Model file for the job. Use its own axes, mm. Face numbers are marked on the shaded views. A direction names the side the tool comes from. Round coordinates to 2 decimals unless told otherwise and drop trailing zeros. Order: outer loops, then holes, each group sorted by start corner. A loop starts at its lowest first (then second) coordinate and runs counter-clockwise, first axis right, second up. Notation, with made-up numbers: (6.25, 82) - (44.25, 82) arc R19 cw to (44.25, 109) - close; hole circle Ø11 at (7.5, 6.5). An arc over 180 degrees is marked (long way). Use one line per item in the form item = value.
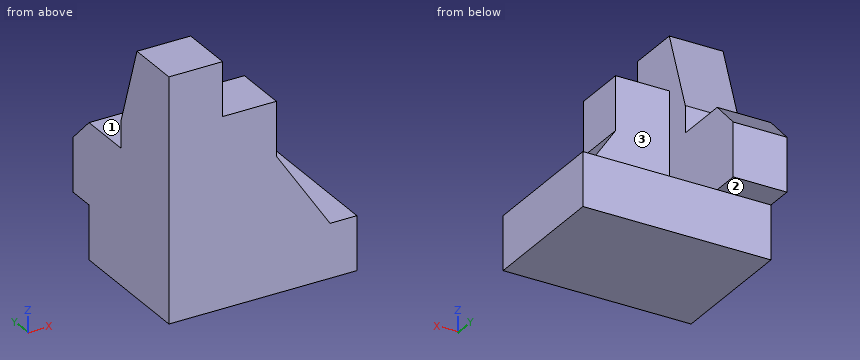
from build123d import *

# Parameters (mm, degrees)
BOSS_EXTRUDE1_DEPTH = 2
BOSS_EXTRUDE2_DEPTH = 3
SKETCH3_W           = 2
SKETCH3_H           = 3
BOSS_EXTRUDE3_DEPTH = 1
CUT_EXTRUDE1_DEPTH  = 3


with BuildPart() as part:
    # Sketch1 → Boss-Extrude1 (new body)
    with BuildSketch(Plane(origin=(0, 0, 0), x_dir=(1, 0, 0), z_dir=(0, 1, 0))):
        Polygon((0, 0), (2, 0), (2, 2), (4, 2), (4, 4), (6, 7), (7, 7), (7, 9), (0, 9), align=None)
    extrude(amount=BOSS_EXTRUDE1_DEPTH)

    # Sketch2 → Boss-Extrude2 (add)
    with BuildSketch(Plane(origin=(0, 2, 0), x_dir=(1, 0, 0), z_dir=(0, 1, 0))):
        Polygon((7, 9), (0, 9), (0, 0), (2, 0), (2, 7), (7, 7), align=None)
    extrude(amount=BOSS_EXTRUDE2_DEPTH)

    # Sketch3 → Boss-Extrude3 (add)
    with BuildSketch(Plane(origin=(0, 5, 0), x_dir=(1, 0, 0), z_dir=(0, 1, 0))):
        with Locations((1, 5.5)):
            Rectangle(SKETCH3_W, SKETCH3_H)
    extrude(amount=BOSS_EXTRUDE3_DEPTH)

    # Sketch4 → Cut-Extrude1 (cut, through all)
    with BuildSketch(Plane(origin=(2, 0, 0), x_dir=(0, 0, -1), z_dir=(1, 0, 0))):
        Polygon((4, 5), (5, 6), (4, 6), align=None)
        Polygon((4, 3), (4, 5), (0, 5), (0, 2), (3, 3), align=None)
    extrude(amount=-CUT_EXTRUDE1_DEPTH, mode=Mode.SUBTRACT)


solid = part.part
(1) Slice it at B-B on x = 2.75. Give the cut face in (y, z).
Report:
outline = (0, -9) - (5, -9) - (5, -7) - (2, -7) - (2, -2) - (0, -2) - close
(2) Slice it at A-A on y = 0.85. Give the cut face in (x, z).
Report:
outline = (0, -9) - (7, -9) - (7, -7) - (6, -7) - (4, -4) - (4, -2) - (2, -2) - (2, 0) - (0, 0) - close
(3) Tool access for the marked faces 1, 2 and 3: list every direction of +Z, -Z, +X, -X, +Y, -Y with a clear straight run to the whole face (end or side of a thin tool).
Report:
face_1 = +Z, +X, -X, +Y
face_2 = -Z, +X, -X, +Y
face_3 = +Z, +X, +Y
(4) Slice it at C-C on z = -3.25. Give the cut face in (x, y).
Report:
outline = (0, 0) - (4, 0) - (4, 2) - (2, 2) - (2, 3) - (0, 3) - close
(5) Pin check, flat tips, straight feed: pin 1 (1.2 mm diameter, centred on x = 4.5, z = -5.5, fed in from +Y); pin 2 (1.6 mm diameter, centred on x = 3, y = 1.5, fed in from +Z); pin 3 (2 mm diameter, centred on x = 5.5, z = -7.5, fed in from -Y); pin 4 (1 mm diameter, centred on y = 0.5, z = -2.5, fed in from +X). Stop position of each tip, or through.
Report:
pin_1 = 2
pin_2 = -2
pin_3 = 0
pin_4 = 4
(6) Probe probe 1 along Z at (x, y) = (6.5, 1.35); probe 2 along X at (y, z) = (3.75, -5.25). List the from-to ranges inside material, lowest first. Write a range as [from, to].
Report:
probe_1 = [-9, -7]
probe_2 = [0, 2]
(7) Slice it at D-D on x = 1.75. Give the cut face in (y, z), then the cut area to 3 significant figures.
Report:
outline = (0, -9) - (5, -9) - (5, -7) - (6, -7) - (6, -5) - (5, -4) - (3, -4) - (3, -3) - (2, 0) - (0, 0) - close
area = 38.0 mm2
